from build123d import *

# Parameters (mm, degrees)
SKETCH1_R           = 17.628998489
BOSS_EXTRUDE1_DEPTH = 6
SKETCH2_R           = 12.777406612
SKETCH2_R_2         = 6.818235005
BOSS_EXTRUDE2_DEPTH = 6
FILLET1_R           = 4.5
FILLET2_R           = 3
DOME1_FACE_RADIUS   = 6.818235005
DOME1_HEIGHT        = 2


with BuildPart() as part:
    # Sketch1 → Boss-Extrude1 (new body)
    with BuildSketch(Plane.XY):
        Circle(SKETCH1_R)
    extrude(amount=BOSS_EXTRUDE1_DEPTH)

    # Sketch2 → Boss-Extrude2 (add)
    with BuildSketch(Plane.XY.offset(6)):
        Circle(SKETCH2_R)
        Circle(SKETCH2_R_2, mode=Mode.SUBTRACT)
    extrude(amount=BOSS_EXTRUDE2_DEPTH)

    # Fillet1
    fillet1_edges = [part.edges().sort_by_distance(p)[0] for p in [
        (-17.628998489, 0, 6),
    ]]
    fillet(fillet1_edges, radius=FILLET1_R)

    # Fillet2
    fillet2_edges = [part.edges().sort_by_distance(p)[0] for p in [
        (-6.818235005, 0, 12),
    ]]
    fillet(fillet2_edges, radius=FILLET2_R)

    # Dome1: a dome of height H over a round flat face of radius A is a cap of a sphere of radius (A * A + H * H) / (2 * H)
    dome1_r = (DOME1_FACE_RADIUS * DOME1_FACE_RADIUS + DOME1_HEIGHT * DOME1_HEIGHT) / (2 * DOME1_HEIGHT)
    dome1_base = Plane((0, 0, 6), z_dir=(0, 0, -1))
    with Locations(dome1_base.offset(DOME1_HEIGHT - dome1_r)):
        dome1_ball = Sphere(dome1_r, mode=Mode.PRIVATE)
    add(split(dome1_ball, bisect_by=dome1_base, keep=Keep.TOP, mode=Mode.PRIVATE), mode=Mode.SUBTRACT)


solid = part.part
Check sheet for the modelled part. Datum: model origin and axes. Units: mm. A direction names the side the tool comes from. Coordinates: 2 decimals unless noted, no trailing zeros. Write each loop counter-clockwise with the first axis right and the second up, starting at its lowest first coordinate (ties: lowest second). Pieces come first, ordered by that corner, then holes. Notation, with made-up numbers: M 7,-11.75 L 31,-11.75 A22 cw 31,-4.75 Z; hole C 9,-15 d8. An arc over 180 degrees is marked long. Answer as CSV lines item,"result".
Q1. Cross-section at D-D (z = 3.5). Record the boundary of the cut face in (x, y).
Check result:
outline,"C 0,0 d34.32"
Q2. Cross-section at A-A (y = 0). Record the boundary of the cut face in (x, z).
Check result:
outline,"M -17.63,0 L 17.63,0 L 17.63,1.5 A4.5 ccw 13.13,6 L 12.78,6 L 12.78,12 L 9.82,12 A3 ccw 6.82,9 L 6.82,6 A12.62 cw -6.82,6 L -6.82,9 A3 ccw -9.82,12 L -12.78,12 L -12.78,6 L -13.13,6 A4.5 ccw -17.63,1.5 Z"
Q3. Set-up check for faces 4 (the face through (0, 0, 0)), 5 (the face through (2.9, -12.6, 6)): record each of +Z, -Z, +X, -X, +Y, -Y from which the full face is reachable in a straight line by a thin tool's end or side.
Check result:
face 4,"-Z, +X, -X, +Y, -Y"
face 5,"+Z"
Q4. Material ranges on probe 1 along Y at (x, z) = (0, 8.45); probe 2 along Z at (x, y) = (5, 12); probe 3 along X at (y, z) = (-2, 7.25), recorded low to high. Write a range as from..to.
Check result:
probe 1,"-12.78..-6.82, 6.82..12.78"
probe 2,"0..6"
probe 3,"-12.62..-6.52, 6.52..12.62"
Q5. Mould release check, pull along Y, two halves, no side actions. Record for faces 1 (the face through (-1.478, -6.656, 7.479)), 2 (the face through (3.7, -9.4, 12)), 3 (the face through (-9.417, 8.636, 8.958)): released by +Y, released by -Y, zero draft, split by the parting line, or undercut.
Check result:
face 1,"undercut"
face 2,"zero draft"
face 3,"split by the parting line"
Q6. Go/stop test with flat-tipped pins: pin 1 (6 mm diameter, centred on x = -7.5, z = 7.5, fed in from +Y); pin 2 (8 mm diameter, centred on x = 0, y = 0, fed in from +Z); pin 3 (4 mm diameter, centred on x = 3.5, z = 11, fed in from +Y). Record where each tip stops, or that it passes through.
Check result:
pin 1,"y = 14.97"
pin 2,"z = 4.65"
pin 3,"y = 12.69"
Q7. Cross-section at C-C (z = 6.75). Record the boundary of the cut face in (x, y), then the cut area to 3 significant figures.
Check result:
outline,"C 0,0 d25.55; hole C 0,0 d13.64"
area,"367 mm^2"
